The model under review builds one solid part; all positions refer to its coordinate system, in mm. A direction names the side the tool comes from. Coordinates: 2 decimals unless noted, no trailing zeros. Write each loop counter-clockwise with the first axis right and the second up, starting at its lowest first coordinate (ties: lowest second). Pieces come first, ordered by that corner, then holes.
1) Machinability: for faces 4 (the cylindrical face through (1.45, 0.07, 1.02)), 5 (the flat face through (6, 6, 2)), 6 (the cylindrical face through (1.951, -7.286, -0.246)), which of the approach directions +Z, -Z, +X, -X, +Y, -Y give a long, thin tool a straight path to every point of the face, cutting with its end or side? Answer none if there is none.
2) For line 1 (Z direction, x = 2.5, y = -11); line 2 (Z direction, x = 2.25, y = -9); line 3 (Y direction, x = 3.5, z = 0.2), list the stretches that pass through material, from the lowest coordinate up.
3) Add section C-C, the plane x = 0. State the section outline as (y, z) points.
4) Add section A-A, the plane x = 3. State the section outline as (y, z) points, then the cut area to 3 significant figures.
5) Mouldability with a two-part tool opening along Y and no side actions: class faces 1 (the cylindrical face through (-1.45, -0.07, 1.02)), 2 (the flat face through (0, 2, -0.5)), 3 (the cylindrical face through (-1.172, 7.423, 2.246)) as released by +Y, released by -Y, zero draft, split by the parting line, or undercut.
6) For P1, Ø1, axis at x = 11, z = 1.5, coming from the -Y side, flat-tipped, find the tip position at first contact; note if it passes through.
7) Add section B-B, the plane y = 0. State the section outline as (x, z) points, then the cut area to 3 significant figures.
8) Add section D-D, the plane z = 0.4. State the section outline as (x, y) points.
from build123d import *

# Parameters (mm, degrees)
SKETCH1_R           = 14
BOSS_EXTRUDE1_DEPTH = 2
SKETCH2_R           = 9
BOSS_EXTRUDE2_DEPTH = 0.5
SKETCH6_R           = 9
BOSS_EXTRUDE4_DEPTH = 0.5
SKETCH7_R           = 1.55
CUT_EXTRUDE1_DEPTH  = 21.024984395


with BuildPart() as part:
    # Sketch1 → Boss-Extrude1 (new body)
    with BuildSketch(Plane.XY):
        Circle(SKETCH1_R)
    extrude(amount=BOSS_EXTRUDE1_DEPTH)

    # Sketch2 → Boss-Extrude2 (add)
    with BuildSketch(Plane.XY.offset(2)):
        with Locations((0, -1.5)):
            Circle(SKETCH2_R)
    extrude(amount=BOSS_EXTRUDE2_DEPTH)

    # Sketch6 → Boss-Extrude4 (add)
    with BuildSketch(Plane(origin=(0, 0, 0), x_dir=(-1, 0, 0), z_dir=(0, 0, -1))):
        with Locations((0, 1.5)):
            Circle(SKETCH6_R)
    extrude(amount=BOSS_EXTRUDE4_DEPTH)

    # Sketch7 → Cut-Extrude1 (cut, through all)
    with BuildSketch(Plane.XY.offset(2.5)):
        with Locations((3, 0)):
            Circle(SKETCH7_R)
        with Locations(Location((-3, 0, 0), (0, 0, 180))):
            Circle(SKETCH7_R)
    extrude(amount=-CUT_EXTRUDE1_DEPTH, mode=Mode.SUBTRACT)


solid = part.part
Geometry results:
1. face 4: +Z, -Z
1. face 5: +Z
1. face 6: -Z
2. line 1: z = 0 to 2
2. line 2: z = 0 to 2.5
2. line 3: y = -13.56 to -1.47, 1.47 to 13.56
3. outline: (-14, 0) - (-7.5, 0) - (-7.5, -0.5) - (10.5, -0.5) - (10.5, 0) - (14, 0) - (14, 2) - (7.5, 2) - (7.5, 2.5) - (-10.5, 2.5) - (-10.5, 2) - (-14, 2) - close
4. outline: (-13.67, 0) - (-6.99, 0) - (-6.99, -0.5) - (-1.55, -0.5) - (-1.55, 2.5) - (-9.99, 2.5) - (-9.99, 2) - (-13.67, 2) - close; (1.55, -0.5) - (9.99, -0.5) - (9.99, 0) - (13.67, 0) - (13.67, 2) - (6.99, 2) - (6.99, 2.5) - (1.55, 2.5) - close
4. area: 62.4 mm2
5. face 1: undercut
5. face 2: zero draft
5. face 3: split by the parting line
6. P1: stops at y = -9.26
7. outline: (-14, 0) - (-8.87, 0) - (-8.87, -0.5) - (-4.55, -0.5) - (-4.55, 2.5) - (-8.87, 2.5) - (-8.87, 2) - (-14, 2) - close; (-1.45, -0.5) - (1.45, -0.5) - (1.45, 2.5) - (-1.45, 2.5) - close; (4.55, -0.5) - (8.87, -0.5) - (8.87, 0) - (14, 0) - (14, 2) - (8.87, 2) - (8.87, 2.5) - (4.55, 2.5) - close
7. area: 55.1 mm2
8. outline: circle Ø28 at (0, 0); hole circle Ø3.1 at (-3, 0); hole circle Ø3.1 at (3, 0)
